Verification items for the finished model (mm, model axes). Face numbers are marked on the shaded views. A direction names the side the tool comes from. Give positions to 0.01 mm unless a question says otherwise; leave off trailing zeros. Order: outer loops, then holes, each group sorted by start corner. A loop starts at its lowest first (then second) coordinate and runs counter-clockwise, first axis right, second up. Notation, with made-up numbers: (85, 40.25) - (99, 40.25) arc R35 ccw to (99, 75.25) - close; hole circle Ø11 at (50.5, 70.5). An arc over 180 degrees is marked (long way). Answer as a JSON object with one key per item and string values. Group by question number.
(1) Section check A-A (z = 0). Record the boundary of the cut face in (x, y), then the cut area to 3 significant figures.
(2) Mould release check, pull along Z, two halves, no side actions. Record for the marked faces 1, 2, 3 and 4: +Z half, -Z half, draft (parallel to the pull), parting line (faces both ways), or undercut.
(3) Depth check by flat-ended pin: pin 1 Ø0.8 at (x, z) = (-0.5, -1) entering from +Y; pin 2 Ø5 at (x, z) = (8, 0) entering from +Y; pin 3 Ø8 at (y, z) = (11.5, 5.5) entering from -X. Enter the tip coordinate at first touch or a pass-through.
(4) Section check B-B (x = 1.25). Record the boundary of the cut face in (y, z).
(5) Section check C-C (y = 5). Record the boundary of the cut face in (x, z), then the cut area to 3 significant figures.
(6) Access from +Z, -Z, +X, -X, +Y, -Y to the whole of each face (thin tool, end or side, straight path). Record for the marked faces 5, 6, 7 and 8.
(7) Thickness scan on line 1 (Z direction, x = 6.25, y = 7.75); line 2 (Y direction, x = 9.75, z = -5). Record the ranges inside material, lowest first.
(8) Section check D-D (x = 16.5). Record the boundary of the cut face in (y, z), then the cut area to 3 significant figures.
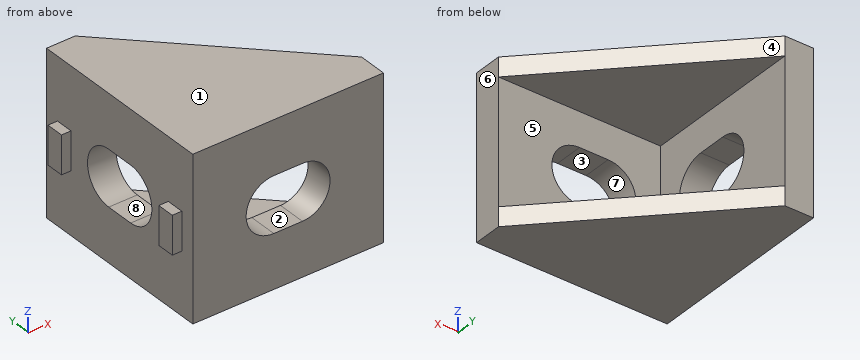
```python
from build123d import *

# Parameters (mm, degrees)
BOSS_EXTRUDE1_DEPTH = 8.5
CUT_EXTRUDE1_START  = -2
CUT_EXTRUDE1_DEPTH  = 13
CUT_EXTRUDE2_DEPTH  = 28.590759323
CUT_EXTRUDE3_DEPTH  = 28.590759323
SKETCH5_W           = 4
SKETCH5_H           = 1.85
BOSS_EXTRUDE2_DEPTH = 1


with BuildPart() as part:
    # Sketch1 → Boss-Extrude1 (new, symmetric)
    with BuildSketch(Plane.XY):
        Polygon((0, 0), (0, 20), (3, 20), (20, 3), (20, 0), align=None)
    extrude(amount=BOSS_EXTRUDE1_DEPTH, both=True)

    # Sketch2 → Cut-Extrude1 (cut)
    with BuildSketch(Plane.XY.offset(8.5).offset(CUT_EXTRUDE1_START)):
        Polygon((3, 20), (3, 3), (20, 3), align=None)
    extrude(amount=-CUT_EXTRUDE1_DEPTH, mode=Mode.SUBTRACT)

    # Sketch3 → Cut-Extrude2 (cut, through all)
    with BuildSketch(Plane(origin=(3, 0, 0), x_dir=(0, 0, -1), z_dir=(1, 0, 0))):
        with BuildLine():
            Line((2.9, 11.5), (2.9, 8.5))
            ThreePointArc((2.9, 8.5), (0, 5.6), (-2.9, 8.5))
            Line((-2.9, 8.5), (-2.9, 11.5))
            ThreePointArc((-2.9, 11.5), (0, 14.4), (2.9, 11.5))
        make_face()
    extrude(amount=-CUT_EXTRUDE2_DEPTH, mode=Mode.SUBTRACT)

    # Sketch4 → Cut-Extrude3 (cut, through all)
    with BuildSketch(Plane(origin=(0, 3, 0), x_dir=(1, 0, 0), z_dir=(0, 1, 0))):
        with BuildLine():
            Line((11.5, -2.9), (8.5, -2.9))
            ThreePointArc((8.5, -2.9), (5.6, 0), (8.5, 2.9))
            Line((8.5, 2.9), (11.5, 2.9))
            ThreePointArc((11.5, 2.9), (14.4, 0), (11.5, -2.9))
        make_face()
    extrude(amount=-CUT_EXTRUDE3_DEPTH, mode=Mode.SUBTRACT)

    # Sketch5 → Boss-Extrude2 (add)
    with BuildSketch(Plane.ZY):
        with Locations((0, 17.575)):
            Rectangle(SKETCH5_W, SKETCH5_H)
        with Locations((0, 2.425)):
            Rectangle(SKETCH5_W, SKETCH5_H)
    extrude(amount=BOSS_EXTRUDE2_DEPTH)


solid = part.part
```
Solutions:
{
 "1": {"outline": "(-1, 1.5) - (0, 1.5) - (0, 0) - (5.6, 0) - (5.6, 3) - (3, 3) - (3, 5.6) - (0, 5.6) - (0, 3.35) - (-1, 3.35) - close; (-1, 16.65) - (0, 16.65) - (0, 14.4) - (3, 14.4) - (3, 20) - (0, 20) - (0, 18.5) - (-1, 18.5) - close; (14.4, 0) - (20, 0) - (20, 3) - (14.4, 3) - close", "area": "61.9 mm2"},
 "2": {"face 1": "+Z half", "face 2": "undercut", "face 3": "undercut", "face 4": "draft"},
 "3": {"pin 1": "stops at y = 18.5", "pin 2": "stops at y = 3", "pin 3": "stops at x = 0"},
 "4": {"outline": "(0, -8.5) - (20, -8.5) - (20, 8.5) - (0, 8.5) - close; hole (8.5, -2.9) - (11.5, -2.9) arc R2.9 ccw to (11.5, 2.9) - (8.5, 2.9) arc R2.9 ccw to start"},
 "5": {"outline": "(0, -8.5) - (18, -8.5) - (18, -6.5) - (3, -6.5) - (3, 6.5) - (18, 6.5) - (18, 8.5) - (0, 8.5) - close", "area": "111 mm2"},
 "6": {"face 5": "+X, +Y", "face 6": "+Z, -Z, +X, +Y, -Y", "face 7": "+Y, -Y", "face 8": "+X, -X"},
 "7": {"line 1": "z = -8.5 to -6.5, 6.5 to 8.5", "line 2": "y = 0 to 3"},
 "8": {"outline": "(0, -8.5) - (6.5, -8.5) - (6.5, -6.5) - (3, -6.5) - (3, 6.5) - (6.5, 6.5) - (6.5, 8.5) - (0, 8.5) - close", "area": "65.0 mm2"}
}
